from build123d import *

# Parameters (mm, degrees)
SKETCH1_W           = 40
SKETCH1_H           = 20
BOSS_EXTRUDE1_DEPTH = 4
SKETCH5_W           = 40
SKETCH5_H           = 4
BOSS_EXTRUDE2_DEPTH = 21
CUT_EXTRUDE3_DEPTH  = 10
CUT_EXTRUDE5_DEPTH  = 10


with BuildPart() as part:
    # Sketch1 → Boss-Extrude1 (new body)
    with BuildSketch(Plane(origin=(0, 0, 0), x_dir=(1, 0, 0), z_dir=(0, 1, 0))):
        with Locations((-29.259259259, 2.888888889)):
            Rectangle(SKETCH1_W, SKETCH1_H)
    extrude(amount=BOSS_EXTRUDE1_DEPTH)

    # Sketch5 → Boss-Extrude2 (add)
    with BuildSketch(Plane(origin=(0, 4, 0), x_dir=(1, 0, 0), z_dir=(0, 1, 0))):
        with Locations((-29.259259259, -5.111111111)):
            Rectangle(SKETCH5_W, SKETCH5_H)
    extrude(amount=BOSS_EXTRUDE2_DEPTH)

    # Sketch7 → Cut-Extrude3 (cut)
    with BuildSketch(Plane(origin=(0, 4, 0), x_dir=(1, 0, 0), z_dir=(0, 1, 0))):
        with BuildLine():
            Line((-15.259259259, 5.588888889), (-43.259259259, 5.588888889))
            ThreePointArc((-43.259259259, 5.588888889), (-45.409259259, 7.738888889), (-43.259259259, 9.888888889))
            Line((-43.259259259, 9.888888889), (-15.259259259, 9.888888889))
            ThreePointArc((-15.259259259, 9.888888889), (-13.109259259, 7.738888889), (-15.259259259, 5.588888889))
        make_face()
    extrude(amount=-CUT_EXTRUDE3_DEPTH, mode=Mode.SUBTRACT)

    # Sketch8 → Cut-Extrude5 (cut)
    with BuildSketch(Plane(origin=(0, 0, 3.111111111), x_dir=(-1, 0, 0), z_dir=(0, 0, -1))):
        with BuildLine():
            Line((24.259259259, 17), (34.259259259, 17))
            ThreePointArc((34.259259259, 17), (36.759259259, 14.5), (34.259259259, 12))
            Line((34.259259259, 12), (24.259259259, 12))
            ThreePointArc((24.259259259, 12), (21.759259259, 14.5), (24.259259259, 17))
        make_face()
    extrude(amount=-CUT_EXTRUDE5_DEPTH, mode=Mode.SUBTRACT)


solid = part.part
CAD build for the part. Positions are in the model's coordinates, mm. A direction names the side the tool comes from. Round coordinates to 2 decimals unless told otherwise and drop trailing zeros. Write each loop counter-clockwise with the first axis right and the second up, starting at its lowest first coordinate (ties: lowest second). Pieces come first, ordered by that corner, then holes. Notation, with made-up numbers: M 42,-0.75 L 100,-0.75 A9 ccw 100,11.25 Z; hole C 71,-29.5 d4. An arc over 180 degrees is marked long. Use a Markdown table: item, result. Add a question column.
1. Flat gauge pins, fed straight in: P1, Ø2, axis at x = -16, z = -0.5, coming from the +Y side; P2, Ø5, axis at y = 14.5, z = -1.5, coming from the -X side; P3, Ø5, axis at x = -13.5, y = 16, coming from the -Z side. Where does each tip first touch, or does it go through?
2. Drill centre lines: probe 1 along Z at (x, y) = (-20.5, 3.75); probe 2 along Z at (x, y) = (-21, 17); probe 3 along Y at (x, z) = (-41, -1). Where is each one in solid material? Low to high.
3. Slice it at C-C on y = 1.5. Give the cut face in (x, z).
4. Slice it at D-D on x = -44. Give the cut face in (y, z), then the cut area to 3 significant figures.
5. Pull direction Y, two halves, no side cores. Call faces 6 (the face through (-30, 25, 5)), 7 (the face through (-45.41, 2.03, -7.69)), 8 (the face through (-30, 0, -1)), 9 (the face through (-29, 12, 5)): released by +Y, released by -Y, zero draft, split by the parting line, or undercut.
6. Slice it at A-A on y = 14.5. Give the cut face in (x, z).
7. Slice it at B-B on z = 5.5. Give the cut face in (x, y), then the cut area to 3 significant figures.
8. 3-axis set-ups, long thin cutter, end or side, ignore diameter. For faces 1 (the face through (-30, 2, -12.889)), 2 (the face through (-29, 2, -9.889)), 3 (the face through (-29, 17, 5)), 4 (the face through (-9.259, 7, 4)), 5 (the face through (-30, 4, -5)): which of +Z, -Z, +X, -X, +Y, -Y reach the whole face in a straight line?
Reply:
| question | item | result |
|---|---|---|
| 1 | P1 | stops at y = 4 |
| 1 | P2 | passes through |
| 1 | P3 | stops at z = 3.11 |
| 2 | probe 1 | z = -12.89 to -9.89, -5.59 to 7.11 |
| 2 | probe 2 | z = 3.11 to 7.11 |
| 2 | probe 3 | y = 0 to 4 |
| 3 | outline | M -49.26,-12.89 L -9.26,-12.89 L -9.26,7.11 L -49.26,7.11 Z; hole M -43.26,-9.89 L -15.26,-9.89 A2.15 ccw -15.26,-5.59 L -43.26,-5.59 A2.15 ccw Z |
| 4 | outline | M 0,-12.89 L 4,-12.89 L 4,-9.76 L 0,-9.76 Z; M 0,-5.72 L 4,-5.72 L 4,3.11 L 25,3.11 L 25,7.11 L 0,7.11 Z |
| 4 | area | 148 mm^2 |
| 5 | face 6 | released by +Y |
| 5 | face 7 | zero draft |
| 5 | face 8 | released by -Y |
| 5 | face 9 | undercut |
| 6 | outline | M -49.26,3.11 L -36.76,3.11 L -36.76,7.11 L -49.26,7.11 Z; M -21.76,3.11 L -9.26,3.11 L -9.26,7.11 L -21.76,7.11 Z |
| 7 | outline | M -49.26,0 L -9.26,0 L -9.26,25 L -49.26,25 Z; hole M -34.26,12 L -24.26,12 A2.5 ccw -24.26,17 L -34.26,17 A2.5 ccw Z |
| 7 | area | 930 mm^2 |
| 8 | face 1 | -Z, +X, -X, +Y, -Y |
| 8 | face 2 | +Y, -Y |
| 8 | face 3 | +Z, -Z |
| 8 | face 4 | +Z, -Z, +X, +Y, -Y |
| 8 | face 5 | -Z, +X, -X, +Y |
